Input: dimensioned drawing with shaded views. Units: mm. Origin: part minimum x, y, z. Give positions to 0.01 mm unless a question says otherwise; leave off trailing zeros. Write each loop counter-clockwise with the first axis right and the second up, starting at its lowest first coordinate (ties: lowest second). Pieces come first, ordered by that corner, then holes. Notation, with made-up numbers: M -21,28.25 L 29,28.25 A36 ccw 29,65.25 Z; hole C 54,47.5 d7. An arc over 180 degrees is marked long. Use CSV: the item, a comma, the result in double quotes. Start each with the question number.
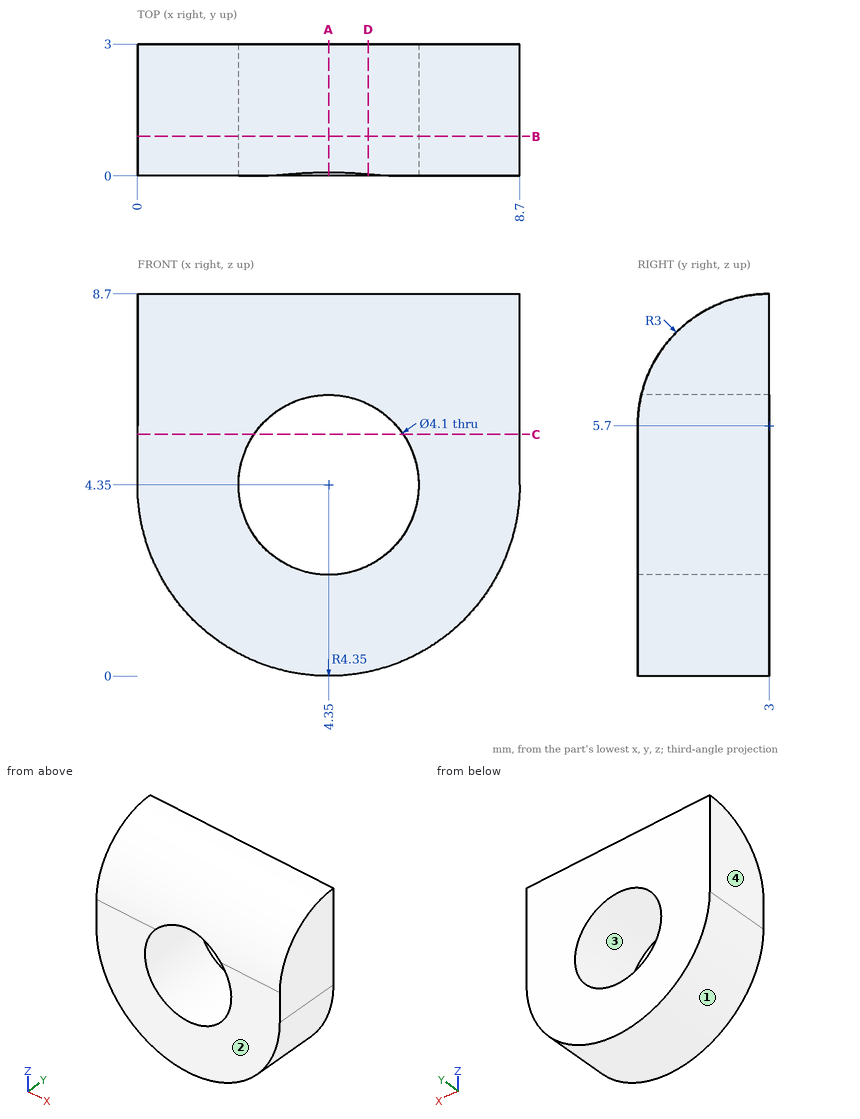
Item 1: Pull-direction query (X, two-part tool) for the marked faces 1, 2, 3 and 4; classes: released by +X, released by -X, zero draft, split by the parting line, or undercut.
Item 2: Section D-D (x = 5.25). Return the cut outline in (y, z), plus the area to 3 significant figures.
Item 3: Section B-B (y = 0.9). Return the cut outline in (x, z), plus the area to 3 significant figures.
Item 4: Material intervals for probe 1 along X at (y, z) = (2.3, 4.35); probe 2 along Z at (x, y) = (4.35, 2.3); probe 3 along Z at (x, y) = (5.25, 1.2), sorted ascending.
Item 5: Section C-C (z = 5.5). Return the cut outline in (x, y).
Item 6: Section A-A (x = 4.35). Return the cut outline in (y, z), plus the area to 3 significant figures.
Output values:
1,face 1,"split by the parting line"
1,face 2,"zero draft"
1,face 3,"undercut"
1,face 4,"released by -X"
2,outline,"M 0,0.09 L 3,0.09 L 3,2.51 L 0,2.51 Z; M 0.04,6.19 L 3,6.19 L 3,8.7 A3 ccw Z"
2,area,"12.8 mm2"
3,outline,"M 0,4.35 A4.35 ccw 8.7,4.35 L 8.7,7.84 L 0,7.84 Z; hole C 4.35,4.35 d4.1"
3,area,"46.9 mm2"
4,probe 1,"x = 0 to 2.3, 6.4 to 8.7"
4,probe 2,"z = 0 to 2.3, 6.4 to 8.62"
4,probe 3,"z = 0.09 to 2.51, 6.19 to 8.1"
5,outline,"M 0,0 L 2.65,0 L 2.65,3 L 0,3 Z; M 6.05,0 L 8.7,0 L 8.7,3 L 6.05,3 Z"
6,outline,"M 0,0 L 3,0 L 3,2.3 L 0,2.3 Z; M 0.08,6.4 L 3,6.4 L 3,8.7 A3 ccw Z"
6,area,"11.9 mm2"
